Build history of the part. All positions in model axes, mm. Round coordinates to 2 decimals unless told otherwise and drop trailing zeros. Write each loop counter-clockwise with the first axis right and the second up, starting at its lowest first coordinate (ties: lowest second). Pieces come first, ordered by that corner, then holes. Notation, with made-up numbers: (26.25, -25.75) -> (55.25, -25.75) arc R20 ccw to (55.25, 8.25) -> close; hole circle Ø6 at (-33.75, 23.5). An arc over 180 degrees is marked (long way). Answer in a Markdown table with one row per item. Add a question column.
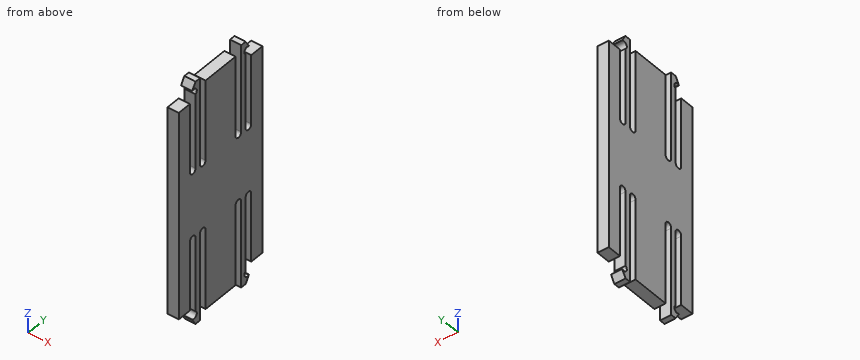
from build123d import *

# Parameters (mm, degrees)
F3_W     = 15
F3_H     = 30
F4_DEPTH = 1.6
F5_W     = 1
F5_H     = 10
F0_DEPTH = 25
F6_W     = 2.7
F6_H     = 1.6
F1_DEPTH = 1.6
F2_R     = 0.5
F7_DEPTH = 25


with BuildPart() as f4:
    # F3 (on Right) → F4 (new body)
    with BuildSketch(Plane.YZ):
        with Locations((7.5, 15)):
            Rectangle(F3_W, F3_H)
    extrude(amount=F4_DEPTH)

    # F5 (on face) → F0 (cut)
    with BuildSketch(Plane.YZ.offset(1.6)):
        with Locations((2.5, 25)):
            Rectangle(F5_W, F5_H)
        with Locations((4.3, 25)):
            Rectangle(F5_W, F5_H)
        with Locations((10.7, 25)):
            Rectangle(F5_W, F5_H)
        with Locations((12.5, 25)):
            Rectangle(F5_W, F5_H)
        with Locations((12.5, 5)):
            Rectangle(F5_W, F5_H)
        with Locations((10.7, 5)):
            Rectangle(F5_W, F5_H)
        with Locations((4.3, 5)):
            Rectangle(F5_W, F5_H)
        with Locations((2.5, 5)):
            Rectangle(F5_W, F5_H)
    extrude(amount=-F0_DEPTH, mode=Mode.SUBTRACT)

    # F6 (on face) → F1 (join)
    with BuildSketch(Plane.YZ.offset(1.6)):
        Polygon((3, 30), (3.8, 30), (3.8, 32.6), (3, 32.6), (2.4, 31.6), (3, 31.6), align=None)
        with Locations((6.15, 30.8)):
            Rectangle(F6_W, F6_H)
        with Locations((8.85, 30.8)):
            Rectangle(F6_W, F6_H)
        Polygon((12, 32.6), (11.2, 32.6), (11.2, 30), (12, 30), (12, 31.6), (12.6, 31.6), align=None)
        Polygon((2.4, -1.6), (3, -2.6), (3.8, -2.6), (3.8, 0), (3, 0), (3, -1.6), align=None)
        Polygon((4.8, 0), (4.8, -1.6), (7.5, -1.6), (10.2, -1.6), (10.2, 0), (7.5, 0), align=None)
        Polygon((12, 0), (11.2, 0), (11.2, -2.6), (12, -2.6), (12.6, -1.6), (12, -1.6), align=None)
    extrude(amount=-F1_DEPTH)

    # F2 (on face) → F7 (cut)
    with BuildSketch(Plane.YZ.offset(1.6)):
        with Locations((4.3, 20)):
            Circle(F2_R)
        with Locations((2.735001, 31.176001)):
            Circle(F2_R)
        with Locations((2.5, 20)):
            Circle(F2_R)
        with Locations((10.7, 20)):
            Circle(F2_R)
        with Locations((12.5, 20)):
            Circle(F2_R)
        with Locations((12.264999, 31.176001)):
            Circle(F2_R)
        with Locations((12.264999, -1.176001)):
            Circle(F2_R)
        with Locations((12.5, 10)):
            Circle(F2_R)
        with Locations((10.7, 10)):
            Circle(F2_R)
        with Locations((4.3, 10)):
            Circle(F2_R)
        with Locations((2.5, 10)):
            Circle(F2_R)
        with Locations((2.735001, -1.176001)):
            Circle(F2_R)
    extrude(amount=-F7_DEPTH, mode=Mode.SUBTRACT)


solid = f4.part
(1) Saw through at C-C (y = 13.5). List the corners of the cut face in (x, z).
(2) Saw through at B-B (y = 9.5). List the corners of the cut face in (x, z).
(3) Saw through at A-A (z = 28). List the corners of the cut face in (x, y), plus the area to 3 significant figures.
(4) Probe line 1 along Y through (x, z) = (1.1, 23); line 2 along Z through (x, y) = (0.65, 8.5); line 3 along Z through (x, y) = (0.15, 1.25). List the from-to ranges inside material, lowest first.
Answer sheet:
| question | item | result |
|---|---|---|
| 1 | outline | (0, 0) -> (1.6, 0) -> (1.6, 30) -> (0, 30) -> close |
| 2 | outline | (0, -1.6) -> (1.6, -1.6) -> (1.6, 31.6) -> (0, 31.6) -> close |
| 3 | outline | (0, 0) -> (1.6, 0) -> (1.6, 2) -> (0, 2) -> close; (0, 3) -> (1.6, 3) -> (1.6, 3.8) -> (0, 3.8) -> close; (0, 4.8) -> (1.6, 4.8) -> (1.6, 10.2) -> (0, 10.2) -> close; (0, 11.2) -> (1.6, 11.2) -> (1.6, 12) -> (0, 12) -> close; (0, 13) -> (1.6, 13) -> (1.6, 15) -> (0, 15) -> close |
| 3 | area | 17.6 mm² |
| 4 | line 1 | y = 0 to 2, 3 to 3.8, 4.8 to 10.2, 11.2 to 12, 13 to 15 |
| 4 | line 2 | z = -1.6 to 31.6 |
| 4 | line 3 | z = 0 to 30 |
